The listing builds one solid part. Answer for the finished solid, in the listing's coordinates (mm). Give positions to 0.01 mm unless a question says otherwise; leave off trailing zeros. Loops run counter-clockwise (first coordinate to the right, second up) from the corner with the lowest first, then second, coordinate; pieces in that order, holes last. Notation, with made-up numbers: M 29.5,30.5 L 35.5,30.5 A20 ccw 35.5,38.5 Z; hole C 68.25,-13 d5. An arc over 180 degrees is marked long. Use one line per item in the form item = value. Start each with the question number.
1. Each of these flat-tipped pins is pushed along its axis until it touches: pin 1 Ø1 at (y, z) = (-2.5, -9.5) entering from +X; pin 2 Ø2 at (x, z) = (2.5, -4.5) entering from +Y; pin 3 Ø1.5 at (y, z) = (-3, -17) entering from -X. Where does it stop, or does it pass through?
2. Straight lines are drawn through the part: line 1 (Y direction, x = 1.25, z = -3); line 2 (Z direction, x = -3.25, y = -1.5) (3 decimals); line 3 (Y direction, x = 1.75, z = -8.25). For each, find the intervals that lie inside material, in ascending order. Write a range as from..to.
3. The part is cut by section A-A (z = -6.75). Write down the section's boundary in (x, y), and give its area (3 significant figures).
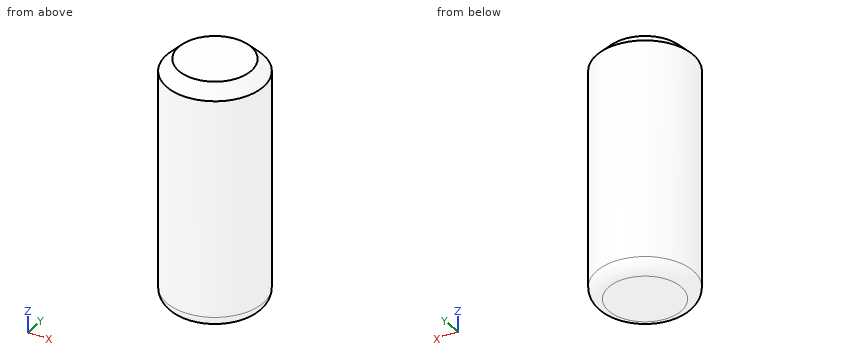
from build123d import *

# Parameters (mm, degrees)
F0_R     = 4
F1_DEPTH = 20
F2_R     = 1
F3_SIZE  = 1


with BuildPart() as f1:
    # F0 (on Top) → F1 (new body)
    with BuildSketch(Plane.XY):
        Circle(F0_R)
    extrude(amount=-F1_DEPTH)

    # F2
    f2_edges = [f1.edges().sort_by_distance(p)[0] for p in [
        (-4, 0, -20),
    ]]
    fillet(f2_edges, radius=F2_R)

    # F3
    f3_edges = [f1.edges().sort_by_distance(p)[0] for p in [
        (-4, 0, 0),
    ]]
    chamfer(f3_edges, length=F3_SIZE)


solid = f1.part
Derived:
q1.pin_1 = 3.46
q1.pin_2 = 3.71
q1.pin_3 = -3.31
q2.line_1 = -3.8..3.8
q2.line_2 = -19.815..-0.579
q2.line_3 = -3.6..3.6
q3.outline = C 0,0 d8
q3.area = 50.3 mm2
